from build123d import *

# Parameters (mm, degrees)
SKETCH1_W                 = 17.78
SKETCH1_H                 = 21.336
BOSS_EXTRUDE1_DEPTH       = 1.3
SKETCH2_W                 = 12
SKETCH2_H                 = 12.5
BOSS_EXTRUDE2_DEPTH       = 2.2
SKETCH4_W                 = 9
SKETCH4_H                 = 7.6
BOSS_EXTRUDE3_DEPTH       = 3.3
CUT_EXTRUDE1_DEPTH        = 2
CUT_EXTRUDE2_DEPTH        = 7.6
FILLET1_R                 = 0.2
FILLET2_R                 = 1.7
SKETCH6_R                 = 0.508
SKETCH6_R_2               = 0.381
CUT_EXTRUDE3_DEPTH        = 2.3
CUT_EXTRUDE4_DEPTH        = 0.05
LPATTERN1_COUNT           = 7
LPATTERN1_PITCH           = 2.54
MIRROR1_COPY_1_SKETCH_R   = 0.508
MIRROR1_COPY_1_SKETCH_R_2 = 0.381
MIRROR1_COPY_1_DEPTH      = 2.3
MIRROR1_COPY_2_SKETCH_R   = 0.508
MIRROR1_COPY_2_SKETCH_R_2 = 0.381
MIRROR1_COPY_2_DEPTH      = 2.3
MIRROR1_COPY_3_SKETCH_R   = 0.508
MIRROR1_COPY_3_SKETCH_R_2 = 0.381
MIRROR1_COPY_3_DEPTH      = 2.3
MIRROR1_COPY_4_SKETCH_R   = 0.508
MIRROR1_COPY_4_SKETCH_R_2 = 0.381
MIRROR1_COPY_4_DEPTH      = 2.3
MIRROR1_COPY_5_SKETCH_R   = 0.508
MIRROR1_COPY_5_SKETCH_R_2 = 0.381
MIRROR1_COPY_5_DEPTH      = 2.3
MIRROR1_COPY_6_SKETCH_R   = 0.508
MIRROR1_COPY_6_SKETCH_R_2 = 0.381
MIRROR1_COPY_6_DEPTH      = 2.3
MIRROR1_COPY_7_DEPTH      = 0.05
MIRROR1_COPY_8_DEPTH      = 0.05
MIRROR1_COPY_9_DEPTH      = 0.05
MIRROR1_COPY_10_DEPTH     = 0.05
MIRROR1_COPY_11_DEPTH     = 0.05
MIRROR1_COPY_12_DEPTH     = 0.05
CUT_EXTRUDE5_DEPTH        = 5


with BuildPart() as part:
    # Sketch1 → Boss-Extrude1 (new body)
    with BuildSketch(Plane(origin=(0, 0, 0), x_dir=(1, 0, 0), z_dir=(0, 1, 0))):
        Rectangle(SKETCH1_W, SKETCH1_H)
    extrude(amount=BOSS_EXTRUDE1_DEPTH)

    # Sketch2 → Boss-Extrude2 (add)
    with BuildSketch(Plane(origin=(0, 1.3, 0), x_dir=(1, 0, 0), z_dir=(0, 1, 0))):
        with Locations((0, -3.118)):
            Rectangle(SKETCH2_W, SKETCH2_H)
    extrude(amount=BOSS_EXTRUDE2_DEPTH)

    # Sketch4 → Boss-Extrude3 (add)
    with BuildSketch(Plane(origin=(0, 1.3, 0), x_dir=(1, 0, 0), z_dir=(0, 1, 0))):
        with Locations((0, 8.268)):
            Rectangle(SKETCH4_W, SKETCH4_H)
    extrude(amount=BOSS_EXTRUDE3_DEPTH)

    # Sketch5 → Cut-Extrude1 (cut)
    with BuildSketch(Plane(origin=(0, 0, -12.068), x_dir=(-1, 0, 0), z_dir=(0, 0, -1))):
        with BuildLine():
            ThreePointArc((-2.85, 1.3), (-4.016726189, 1.783273811), (-4.5, 2.95))
            Line((-4.5, 2.95), (-4.5, 1.3))
            Line((-4.5, 1.3), (-2.85, 1.3))
        make_face()
        with BuildLine():
            Line((4.5, 1.3), (4.5, 2.95))
            ThreePointArc((4.5, 2.95), (4.016726189, 1.783273811), (2.85, 1.3))
            Line((2.85, 1.3), (4.5, 1.3))
        make_face()
    extrude(amount=-CUT_EXTRUDE1_DEPTH, mode=Mode.SUBTRACT)

    # Sketch5<3> → Cut-Extrude2 (cut)
    with BuildSketch(Plane(origin=(0, 0, -12.068), x_dir=(-1, 0, 0), z_dir=(0, 0, -1))):
        with BuildLine():
            Line((4.5, 4.6), (2.85, 4.6))
            ThreePointArc((2.85, 4.6), (4.016726189, 4.116726189), (4.5, 2.95))
            Line((4.5, 2.95), (4.5, 4.6))
        make_face()
        with BuildLine():
            ThreePointArc((-4.5, 2.95), (-4.016726189, 4.116726189), (-2.85, 4.6))
            Line((-2.85, 4.6), (-4.5, 4.6))
            Line((-4.5, 4.6), (-4.5, 2.95))
        make_face()
    extrude(amount=-CUT_EXTRUDE2_DEPTH, mode=Mode.SUBTRACT)

    # Fillet1
    fillet1_edges = [part.edges().sort_by_distance(p)[0] for p in [
        (6, 2.4, 9.368),
        (6, 2.4, -3.132),
        (-6, 2.4, -3.132),
        (-6, 2.4, 9.368),
        (6, 3.5, 3.118),
        (0, 3.5, -3.132),
        (-6, 3.5, 3.118),
        (0, 3.5, 9.368),
    ]]
    fillet(fillet1_edges, radius=FILLET1_R)

    # Fillet2
    fillet2_edges = [part.edges().sort_by_distance(p)[0] for p in [
        (-8.89, 0.65, -10.668),
        (8.89, 0.65, -10.668),
        (8.89, 0.65, 10.668),
        (-8.89, 0.65, 10.668),
    ]]
    fillet(fillet2_edges, radius=FILLET2_R)

    # Sketch6 → Cut-Extrude3 (cut, through all)
    with BuildSketch(Plane(origin=(0, 1.3, 0), x_dir=(1, 0, 0), z_dir=(0, 1, 0))):
        with Locations((-7.62, 7.62)):
            Circle(SKETCH6_R)
        with Locations((-8.89, 7.62)):
            Circle(SKETCH6_R_2)
    cut_extrude3 = extrude(amount=-CUT_EXTRUDE3_DEPTH, mode=Mode.SUBTRACT)

    # Sketch7 → Cut-Extrude4 (cut)
    with BuildSketch(Plane(origin=(0, 1.3, 0), x_dir=(1, 0, 0), z_dir=(0, 1, 0))):
        with BuildLine():
            Line((-8.89, 8.528), (-7.62, 8.528))
            ThreePointArc((-7.62, 8.528), (-6.712, 7.62), (-7.62, 6.712))
            Line((-7.62, 6.712), (-8.89, 6.712))
            Line((-8.89, 6.712), (-8.89, 8.528))
        make_face()
    cut_extrude4 = extrude(amount=-CUT_EXTRUDE4_DEPTH, mode=Mode.SUBTRACT)

    # LPattern1: Cut-Extrude3, Cut-Extrude4 ×7
    with Locations(*[(0, 0, i * LPATTERN1_PITCH) for i in range(1, LPATTERN1_COUNT)]):
        add(cut_extrude3, mode=Mode.SUBTRACT)
        add(cut_extrude4, mode=Mode.SUBTRACT)

    # Mirror1: Cut-Extrude3, Cut-Extrude4 across plane
    add(cut_extrude3.mirror(Plane(origin=(0, 0, 0), x_dir=(0, 0, 1), z_dir=(1, 0, 0))), mode=Mode.SUBTRACT)
    add(cut_extrude4.mirror(Plane(origin=(0, 0, 0), x_dir=(0, 0, 1), z_dir=(1, 0, 0))), mode=Mode.SUBTRACT)

    # Mirror1 copy 1 sketch → Mirror1 copy 1 (cut, through all)
    with BuildSketch(Plane(origin=(0, 1.3, 2.54), x_dir=(-1, 0, 0), z_dir=(0, 1, 0))):
        with Locations((-7.62, -7.62)):
            Circle(MIRROR1_COPY_1_SKETCH_R)
        with Locations((-8.89, -7.62)):
            Circle(MIRROR1_COPY_1_SKETCH_R_2)
    extrude(amount=-MIRROR1_COPY_1_DEPTH, mode=Mode.SUBTRACT)

    # Mirror1 copy 2 sketch → Mirror1 copy 2 (cut, through all)
    with BuildSketch(Plane(origin=(0, 1.3, 5.08), x_dir=(-1, 0, 0), z_dir=(0, 1, 0))):
        with Locations((-7.62, -7.62)):
            Circle(MIRROR1_COPY_2_SKETCH_R)
        with Locations((-8.89, -7.62)):
            Circle(MIRROR1_COPY_2_SKETCH_R_2)
    extrude(amount=-MIRROR1_COPY_2_DEPTH, mode=Mode.SUBTRACT)

    # Mirror1 copy 3 sketch → Mirror1 copy 3 (cut, through all)
    with BuildSketch(Plane(origin=(0, 1.3, 7.62), x_dir=(-1, 0, 0), z_dir=(0, 1, 0))):
        with Locations((-7.62, -7.62)):
            Circle(MIRROR1_COPY_3_SKETCH_R)
        with Locations((-8.89, -7.62)):
            Circle(MIRROR1_COPY_3_SKETCH_R_2)
    extrude(amount=-MIRROR1_COPY_3_DEPTH, mode=Mode.SUBTRACT)

    # Mirror1 copy 4 sketch → Mirror1 copy 4 (cut, through all)
    with BuildSketch(Plane(origin=(0, 1.3, 10.16), x_dir=(-1, 0, 0), z_dir=(0, 1, 0))):
        with Locations((-7.62, -7.62)):
            Circle(MIRROR1_COPY_4_SKETCH_R)
        with Locations((-8.89, -7.62)):
            Circle(MIRROR1_COPY_4_SKETCH_R_2)
    extrude(amount=-MIRROR1_COPY_4_DEPTH, mode=Mode.SUBTRACT)

    # Mirror1 copy 5 sketch → Mirror1 copy 5 (cut, through all)
    with BuildSketch(Plane(origin=(0, 1.3, 12.7), x_dir=(-1, 0, 0), z_dir=(0, 1, 0))):
        with Locations((-7.62, -7.62)):
            Circle(MIRROR1_COPY_5_SKETCH_R)
        with Locations((-8.89, -7.62)):
            Circle(MIRROR1_COPY_5_SKETCH_R_2)
    extrude(amount=-MIRROR1_COPY_5_DEPTH, mode=Mode.SUBTRACT)

    # Mirror1 copy 6 sketch → Mirror1 copy 6 (cut, through all)
    with BuildSketch(Plane(origin=(0, 1.3, 15.24), x_dir=(-1, 0, 0), z_dir=(0, 1, 0))):
        with Locations((-7.62, -7.62)):
            Circle(MIRROR1_COPY_6_SKETCH_R)
        with Locations((-8.89, -7.62)):
            Circle(MIRROR1_COPY_6_SKETCH_R_2)
    extrude(amount=-MIRROR1_COPY_6_DEPTH, mode=Mode.SUBTRACT)

    # Mirror1 copy 7 sketch → Mirror1 copy 7 (cut)
    with BuildSketch(Plane(origin=(0, 1.3, 2.54), x_dir=(-1, 0, 0), z_dir=(0, 1, 0))):
        with BuildLine():
            Line((-8.89, -8.528), (-7.62, -8.528))
            ThreePointArc((-7.62, -8.528), (-6.712, -7.62), (-7.62, -6.712))
            Line((-7.62, -6.712), (-8.89, -6.712))
            Line((-8.89, -6.712), (-8.89, -8.528))
        make_face()
    extrude(amount=-MIRROR1_COPY_7_DEPTH, mode=Mode.SUBTRACT)

    # Mirror1 copy 8 sketch → Mirror1 copy 8 (cut)
    with BuildSketch(Plane(origin=(0, 1.3, 5.08), x_dir=(-1, 0, 0), z_dir=(0, 1, 0))):
        with BuildLine():
            Line((-8.89, -8.528), (-7.62, -8.528))
            ThreePointArc((-7.62, -8.528), (-6.712, -7.62), (-7.62, -6.712))
            Line((-7.62, -6.712), (-8.89, -6.712))
            Line((-8.89, -6.712), (-8.89, -8.528))
        make_face()
    extrude(amount=-MIRROR1_COPY_8_DEPTH, mode=Mode.SUBTRACT)

    # Mirror1 copy 9 sketch → Mirror1 copy 9 (cut)
    with BuildSketch(Plane(origin=(0, 1.3, 7.62), x_dir=(-1, 0, 0), z_dir=(0, 1, 0))):
        with BuildLine():
            Line((-8.89, -8.528), (-7.62, -8.528))
            ThreePointArc((-7.62, -8.528), (-6.712, -7.62), (-7.62, -6.712))
            Line((-7.62, -6.712), (-8.89, -6.712))
            Line((-8.89, -6.712), (-8.89, -8.528))
        make_face()
    extrude(amount=-MIRROR1_COPY_9_DEPTH, mode=Mode.SUBTRACT)

    # Mirror1 copy 10 sketch → Mirror1 copy 10 (cut)
    with BuildSketch(Plane(origin=(0, 1.3, 10.16), x_dir=(-1, 0, 0), z_dir=(0, 1, 0))):
        with BuildLine():
            Line((-8.89, -8.528), (-7.62, -8.528))
            ThreePointArc((-7.62, -8.528), (-6.712, -7.62), (-7.62, -6.712))
            Line((-7.62, -6.712), (-8.89, -6.712))
            Line((-8.89, -6.712), (-8.89, -8.528))
        make_face()
    extrude(amount=-MIRROR1_COPY_10_DEPTH, mode=Mode.SUBTRACT)

    # Mirror1 copy 11 sketch → Mirror1 copy 11 (cut)
    with BuildSketch(Plane(origin=(0, 1.3, 12.7), x_dir=(-1, 0, 0), z_dir=(0, 1, 0))):
        with BuildLine():
            Line((-8.89, -8.528), (-7.62, -8.528))
            ThreePointArc((-7.62, -8.528), (-6.712, -7.62), (-7.62, -6.712))
            Line((-7.62, -6.712), (-8.89, -6.712))
            Line((-8.89, -6.712), (-8.89, -8.528))
        make_face()
    extrude(amount=-MIRROR1_COPY_11_DEPTH, mode=Mode.SUBTRACT)

    # Mirror1 copy 12 sketch → Mirror1 copy 12 (cut)
    with BuildSketch(Plane(origin=(0, 1.3, 15.24), x_dir=(-1, 0, 0), z_dir=(0, 1, 0))):
        with BuildLine():
            Line((-8.89, -8.528), (-7.62, -8.528))
            ThreePointArc((-7.62, -8.528), (-6.712, -7.62), (-7.62, -6.712))
            Line((-7.62, -6.712), (-8.89, -6.712))
            Line((-8.89, -6.712), (-8.89, -8.528))
        make_face()
    extrude(amount=-MIRROR1_COPY_12_DEPTH, mode=Mode.SUBTRACT)

    # Sketch8 → Cut-Extrude5 (cut)
    with BuildSketch(Plane(origin=(0, 0, -12.068), x_dir=(-1, 0, 0), z_dir=(0, 0, -1))):
        with BuildLine():
            Line((2.85, 4.4), (-2.85, 4.4))
            ThreePointArc((-2.85, 4.4), (-4.3, 2.95), (-2.85, 1.5))
            Line((-2.85, 1.5), (2.85, 1.5))
            ThreePointArc((2.85, 1.5), (4.3, 2.95), (2.85, 4.4))
        make_face()
    extrude(amount=-CUT_EXTRUDE5_DEPTH, mode=Mode.SUBTRACT)


solid = part.part
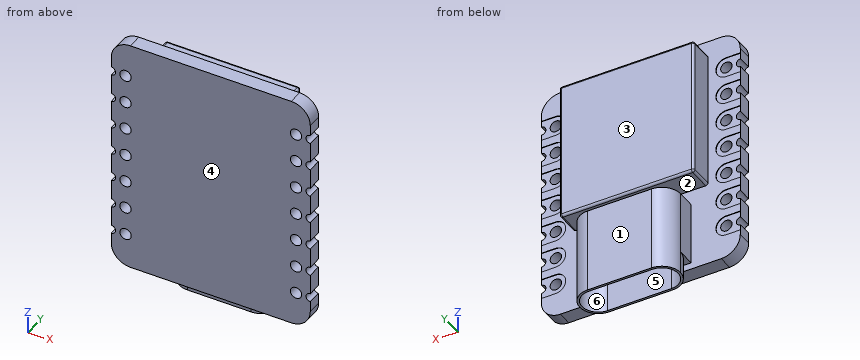
Build history of the part. All positions in model axes, mm. Face numbers are marked on the shaded views. A direction names the side the tool comes from. Round coordinates to 2 decimals unless told otherwise and drop trailing zeros. Write each loop counter-clockwise with the first axis right and the second up, starting at its lowest first coordinate (ties: lowest second). Pieces come first, ordered by that corner, then holes. Notation, with made-up numbers: (73, 67) - (102, 67) arc R18 ccw to (102, 83) - close; hole circle Ø8 at (18, -1). An arc over 180 degrees is marked (long way). Use CSV: the item, a comma, the result in double quotes.
(1) Mould opens along X. For the marked faces 4, 5 and 6 say: pulls with the +X half, pulls with the -X half, needs draft (parallel to the pull), parting line crosses it, or undercut.
Response:
face 4,"needs draft"
face 5,"undercut"
face 6,"undercut"
(2) 3-axis set-ups, long thin cutter, end or side, ignore diameter. For the marked faces 1, 2 and 3: which of +Z, -Z, +X, -X, +Y, -Y reach the whole face in a straight line?
Response:
face 1,"+Z, -Z, +X, -X, +Y"
face 2,"+X, -X, +Y"
face 3,"+Z, +X, -X, +Y"
(3) Pin check, flat tips, straight feed: P1, Ø1, axis at x = 1.5, y = 2.5, coming from the -Z side; P2, Ø1.2, axis at x = 7.62, z = -5.08, coming from the -Y side; P3, Ø3.5, axis at x = -1, z = 5.5, coming from the +Y side; P4, Ø2, axis at x = -8, z = 7.5, coming from the +Y side. Stop position of each tip, or through.
Response:
P1,"z = -7.07"
P2,"y = 0"
P3,"y = 3.5"
P4,"y = 1.3"
(4) Wall check: line 1 (Y direction, x = -1.75, z = -8.5); line 2 (Z direction, x = 3.25, y = 2.25); line 3 (Y direction, x = 5, z = -8). Give the ranges that are in metal, low to high.
Response:
line 1,"0 to 1.5, 4.4 to 4.6"
line 2,"-7.07 to -4.47, -3.13 to 9.37"
line 3,"0 to 1.3"
(5) Band-saw the part on B-B (y = 2.15). Write the cut outline in (x, z).
Response:
outline,"(-6, -2.93) arc R0.2 ccw to (-5.8, -3.13) - (5.8, -3.13) arc R0.2 ccw to (6, -2.93) - (6, 9.17) arc R0.2 ccw to (5.8, 9.37) - (-5.8, 9.37) arc R0.2 ccw to (-6, 9.17) - close; (-4.5, -10.07) - (-4.29, -10.07) - (-4.29, -12.07) - (-4.06, -12.07) - (-4.06, -7.07) - (4.06, -7.07) - (4.06, -12.07) - (4.29, -12.07) - (4.29, -10.07) - (4.5, -10.07) - (4.5, -4.47) - (-4.5, -4.47) - close"
(6) Band-saw the part on A-A (z = 5.08). Write the cut outline in (x, y), plus the area to 3 significant figures.
Response:
outline,"(-8.51, 0) - (-8.13, 0) - (-8.13, 1.25) - (-8.51, 1.25) - close; (-7.11, 0) - (7.11, 0) - (7.11, 1.25) - (6.71, 1.25) - (6.71, 1.3) - (6, 1.3) - (6, 3.3) arc R0.2 ccw to (5.8, 3.5) - (-5.8, 3.5) arc R0.2 ccw to (-6, 3.3) - (-6, 1.3) - (-6.71, 1.3) - (-6.71, 1.25) - (-7.11, 1.25) - close; (8.13, 0) - (8.51, 0) - (8.51, 1.25) - (8.13, 1.25) - close"
area,"45.8 mm²"
(7) Band-saw the part on C-C (x = -1.5). Write the cut outline in (y, z), plus the area to 3 significant figures.
Response:
outline,"(0, -10.67) - (1.3, -10.67) - (1.3, -12.07) - (1.5, -12.07) - (1.5, -7.07) - (4.4, -7.07) - (4.4, -12.07) - (4.6, -12.07) - (4.6, -4.47) - (1.3, -4.47) - (1.3, -3.13) - (3.3, -3.13) arc R0.2 ccw to (3.5, -2.93) - (3.5, 9.17) arc R0.2 ccw to (3.3, 9.37) - (1.3, 9.37) - (1.3, 10.67) - (0, 10.67) - close"
area,"65.8 mm²"
(8) Band-saw the part on D-D (y = 0.6). Give the number of separate pieces and of enclosed holes in the cut face, plus the area to 3 significant figures.
Response:
separate pieces,"1"
enclosed holes,"14"
area,"362 mm²"
